from build123d import *

# Parameters (mm, degrees)
F2_R     = 29.21
F2_R_2   = 25.4
F3_DEPTH = 25.4
F4_DEPTH = 25.4
F5_R     = 29.21
F6_DEPTH = 38.1
F7_DEPTH = 50.8
F8_R     = 10.16


with BuildPart() as f1:
    # F0 (on Front) → F1 (revolve)
    with BuildSketch(Plane.XZ):
        Polygon((25.4, 0), (0, 0), (0, -75.989135), (0, -304.8), (25.4, -304.8), align=None)
    revolve(axis=Axis((0, 0, -37.994567), (0, 0, -1)))

    # F2 (on Top) → F3 (join)
    with BuildSketch(Plane.XY):
        Circle(F2_R)
        Circle(F2_R_2, mode=Mode.SUBTRACT)
    extrude(amount=-F3_DEPTH)

    # F2 (on Top) → F4 (join)
    with BuildSketch(Plane.XY):
        Circle(F2_R)
        Circle(F2_R_2, mode=Mode.SUBTRACT)
    extrude(amount=F4_DEPTH)

    # F5 (on Right) → F6 (cut, symmetric)
    with BuildSketch(Plane.YZ):
        with Locations((0, 33.02)):
            Circle(F5_R)
    extrude(amount=F6_DEPTH, both=True, mode=Mode.SUBTRACT)

    # F5 (on Right) → F7 (join, symmetric)
    with BuildSketch(Plane.YZ):
        with Locations((0, 33.02)):
            Circle(F5_R)
    extrude(amount=F7_DEPTH, both=True)

    # F8
    f8_edges = [f1.edges().sort_by_distance(p)[0] for p in [
        (-25.4, 0, -304.8),
    ]]
    fillet(f8_edges, radius=F8_R)


solid = f1.part
Read the model definition and answer for the solid it produces. Units are mm, in the model's axes. A direction names the side the tool comes from. Coordinates: 2 decimals unless noted, no trailing zeros. Write each loop counter-clockwise with the first axis right and the second up, starting at its lowest first coordinate (ties: lowest second). Pieces come first, ordered by that corner, then holes. Notation, with made-up numbers: M 84.25,76 L 114.25,76 A17 cw 114.25,109 Z; hole C 73.5,5.5 d3. An arc over 180 degrees is marked long. Use a Markdown table: item, result.
Q1. Each of these flat-tipped pins is pushed along its axis until it touches: pin 1 Ø10 at (x, y) = (31, -1) entering from +Z; pin 2 Ø8 at (y, z) = (16.5, -45.5) entering from -X; pin 3 Ø1.5 at (y, z) = (0.5, -159.5) entering from +X; pin 4 Ø3 at (x, z) = (-27.5, -102.5) entering from -Y. Where does it stop, or does it pass through?
Answer block:
| item | result |
|---|---|
| pin 1 | stops at z = 62.23 |
| pin 2 | stops at x = -22.11 |
| pin 3 | stops at x = 25.4 |
| pin 4 | passes through |
Q2. Straight lines are drawn through the part: L1, parallel to Y at x = 0, z = 8; L2, parallel to Y at x = 14, z = 33.5; L3, parallel to Z at x = -17, y = 15. For each, find the intervals that lie inside material, in ascending order. Write a range as [from, to].
Answer block:
| item | result |
|---|---|
| L1 | y = [-29.21, -25.4], [-15.07, 15.07], [25.4, 29.21] |
| L2 | y = [-29.21, 29.21] |
| L3 | z = [-301.57, 0], [7.96, 58.08] |
Q3. The part is cut by section B-B, the plane y = 0. Write down the section's boundary in (x, z), then the cut area to 3 significant figures.
Answer block:
| item | result |
|---|---|
| outline | M -50.8,3.81 L -29.21,3.81 L -29.21,-25.4 L -25.4,-25.4 L -25.4,-294.64 A10.16 ccw -15.24,-304.8 L 15.24,-304.8 A10.16 ccw 25.4,-294.64 L 25.4,-25.4 L 29.21,-25.4 L 29.21,3.81 L 50.8,3.81 L 50.8,62.23 L -50.8,62.23 Z; hole M -25.4,0 L 25.4,0 L 25.4,3.81 L -25.4,3.81 Z |
| area | 21,600 mm2 |
Q4. Determine the mould class of faces 1 (the face through (-5.506, 24.796, -158.135)), 2 (the face through (0, 0, 0)), 3 (the face through (50.8, 0, 33)) for opening direction Y: released by +Y, released by -Y, zero draft, split by the parting line, or undercut.
Answer block:
| item | result |
|---|---|
| face 1 | split by the parting line |
| face 2 | undercut |
| face 3 | zero draft |
Q5. Which of the six approach directions +Z, -Z, +X, -X, +Y, -Y give full straight-line access (tool end or side, diameter ignored) to faces 4 (the face through (-50.8, 0, 33)), 5 (the face through (-20.157, -15.456, 7.101)), 6 (the face through (-9, 24, -25.4))?
Answer block:
| item | result |
|---|---|
| face 4 | +Z, -Z, -X, +Y, -Y |
| face 5 | none |
| face 6 | -Z |
Q6. The part is cut by section C-C, the plane z = -87. Write down the section's boundary in (x, y).
Answer block:
| item | result |
|---|---|
| outline | C 0,0 d50.8 |
Q7. The part is cut by section D-D, the plane x = -42.5. Write down the section's boundary in (y, z).
Answer block:
| item | result |
|---|---|
| outline | C 0,33.02 d58.42 |
Q8. The part is cut by section A-A, the plane x = 0. Write down the section's boundary in (y, z), then the cut area to 3 significant figures.
Answer block:
| item | result |
|---|---|
| outline | M -29.21,-25.4 L -25.4,-25.4 L -25.4,-294.64 A10.16 ccw -15.24,-304.8 L 15.24,-304.8 A10.16 ccw 25.4,-294.64 L 25.4,-25.4 L 29.21,-25.4 L 29.21,25.4 L 28.2,25.4 A29.21 ccw long -28.2,25.4 L -29.21,25.4 Z; hole M -25.4,0 L 25.4,0 L 25.4,18.6 A29.21 cw -25.4,18.6 Z |
| area | 18,500 mm2 |
